Design review of the part built by this model. Coordinates are the model's own, in mm. Face numbers are marked on the shaded views. Coordinates: 2 decimals unless noted, no trailing zeros. Order: outer loops, then holes, each group sorted by start corner. A loop starts at its lowest first (then second) coordinate and runs counter-clockwise, first axis right, second up. Notation, with made-up numbers: (65, 33.5) -> (99, 33.5) arc R21 ccw to (99, 50.5) -> close; hole circle Ø2 at (71, 14). An arc over 180 degrees is marked (long way). Write item = value, one per line.
```python
from build123d import *

# Parameters (mm, degrees)
CROQUIS1_W                = 22
CROQUIS1_H                = 22
CROQUIS1_R                = 9.25
SALIENTE_EXTRUIR1_DEPTH   = 70
REDONDEO1_R               = 11
CROQUIS6_W                = 22
CROQUIS6_H                = 70
SALIENTE_EXTRUIR2_DEPTH   = 3
TALADRO_ROSCADO_M51_D     = 4.2
TALADRO_ROSCADO_M51_DEPTH = 14
TALADRO_ROSCADO_M51_TIP   = 1.2618073


with BuildPart() as part:
    # Croquis1 → Saliente-Extruir1 (new body)
    with BuildSketch(Plane.XY):
        with Locations((11, -11)):
            Rectangle(CROQUIS1_W, CROQUIS1_H)
        with Locations((11, -11)):
            Circle(CROQUIS1_R, mode=Mode.SUBTRACT)
    extrude(amount=SALIENTE_EXTRUIR1_DEPTH)

    # Redondeo1
    redondeo1_edges = [part.edges().sort_by_distance(p)[0] for p in [
        (22, 0, 35),
        (0, 0, 35),
    ]]
    fillet(redondeo1_edges, radius=REDONDEO1_R - 0.0001)  # a hair under: the kernel refuses the full size

    # Croquis6 → Saliente-Extruir2 (add)
    with BuildSketch(Plane.XZ.offset(22)):
        with Locations((11, 35)):
            Rectangle(CROQUIS6_W, CROQUIS6_H)
    extrude(amount=SALIENTE_EXTRUIR2_DEPTH)

    # Taladro roscado M51
    with Locations(Plane(origin=(0, -25, 0), x_dir=(-1, 0, 0), z_dir=(0, -1, 0))):
        with Locations((-11, -7.622118599), (-11, -17.622118599), (-11, -27.622118599)):
            Hole(TALADRO_ROSCADO_M51_D / 2, depth=TALADRO_ROSCADO_M51_DEPTH)
            with Locations((0, 0, -(TALADRO_ROSCADO_M51_DEPTH + TALADRO_ROSCADO_M51_TIP / 2))):  # 118° drill point
                Cone(0, TALADRO_ROSCADO_M51_D / 2, TALADRO_ROSCADO_M51_TIP, mode=Mode.SUBTRACT)


solid = part.part
```
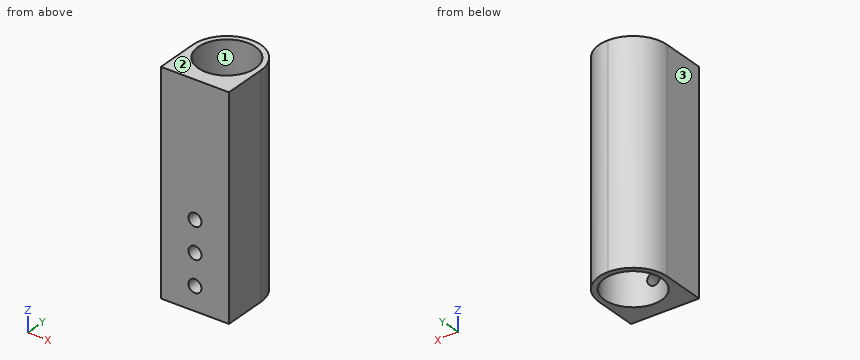
(1) We need section D-D (x = 10). Write out the cut boundary in (y, z), and give its area (3 significant figures).
Report:
outline = (-25, 0) -> (-20.2, 0) -> (-20.2, 5.78) -> (-25, 5.78) -> close; (-25, 9.47) -> (-20.2, 9.47) -> (-20.2, 15.78) -> (-25, 15.78) -> close; (-25, 19.47) -> (-20.2, 19.47) -> (-20.2, 25.78) -> (-25, 25.78) -> close; (-25, 29.47) -> (-20.2, 29.47) -> (-20.2, 70) -> (-25, 70) -> close; (-1.8, 0) -> (-0.05, 0) -> (-0.05, 70) -> (-1.8, 70) -> close
area = 406 mm²
(2) We need section B-B (y = -12). Write out the cut boundary in (x, z).
Report:
outline = (0, 0) -> (1.8, 0) -> (1.8, 70) -> (0, 70) -> close; (20.2, 0) -> (22, 0) -> (22, 70) -> (20.2, 70) -> close
(3) Insertion check: pin 1 (3.5 mm diameter, centred on x = 11, z = 7.62, fed in from -Y); pin 2 (2 mm diameter, centred on y = -4, z = 43.5, fed in from -X); pin 3 (3 mm diameter, centred on x = 4.5, z = 41.5, fed in from +Y). Each pin has a flat end and moves straight along its axis. Give the tip position at first contact, or say it passes through.
Report:
pin_1 = -1.92
pin_2 = 1.78
pin_3 = -1.2
(4) For L1, parallel to Z at x = 11, y = -21.4; L2, parallel to X at y = -8.5, z = 35; L3, parallel to X at y = -18.25, z = 33.5, list the stretches that pass through material, from the lowest coordinate up.
Report:
L1 = 0 to 5.52, 9.72 to 15.52, 19.72 to 25.52, 29.72 to 70
L2 = 0.29 to 2.09, 19.91 to 21.71
L3 = 0 to 5.26, 16.74 to 22
(5) We need section C-C (x = 3.25). Write out the cut boundary in (y, z).
Report:
outline = (-25, 0) -> (-16.05, 0) -> (-16.05, 70) -> (-25, 70) -> close; (-5.95, 0) -> (-3.19, 0) -> (-3.19, 70) -> (-5.95, 70) -> close
(6) The part is to be moulded in two halves that separate along X. For the marked faces 1, 2 and 3, say which applies: released by +X, released by -X, zero draft, split by the parting line, or undercut.
Report:
face_1 = undercut
face_2 = zero draft
face_3 = released by -X
